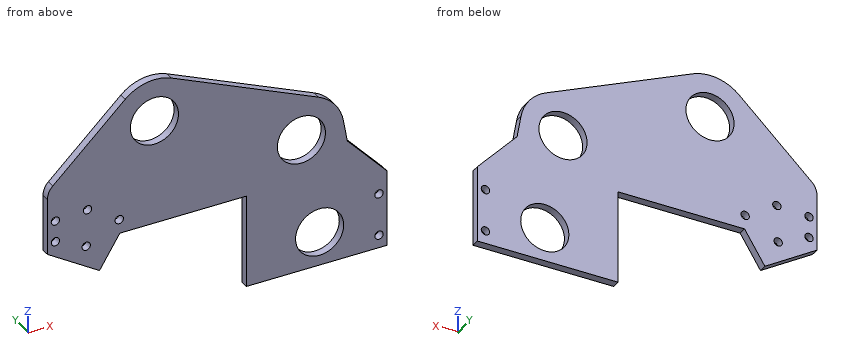
from build123d import *

# Parameters (mm, degrees)
SKETCH1_R              = 14.29004
BOSS_EXTRUDE1_DEPTH    = 4.7625
FILLET1_R              = 10
F_10_CLEARANCE_HOLE1_D = 4.9784
F_10_CLEARANCE_HOLE2_D = 4.9784


with BuildPart() as part:
    # Sketch1 → Boss-Extrude1 (new body)
    with BuildSketch(Plane(origin=(0, 0, 0), x_dir=(1, 0, 0), z_dir=(0, 1, 0))):
        with BuildLine():
            Line((-62.06952, -79.895280222), (25.163028109, -41.695780276))
            ThreePointArc((25.163028109, -41.695780276), (34.911191298, -34.148496119), (39.936134607, -22.890693115))
            Line((39.936134607, -22.890693115), (42.271095404, -9.586739751))
            Line((42.271095404, -9.586739751), (65.82695514, 16.012754812))
            Line((65.82695514, 16.012754812), (65.826833771, 61.726825209))
            Line((65.826833771, 61.726825209), (-17.734439664, 61.726825209))
            Line((-17.734439664, 61.726825209), (-17.734439664, 6.164245545))
            Line((-17.734439664, 6.164245545), (-92.776319002, 6.164245545))
            Line((-92.776319002, 6.164245545), (-104.854054452, 25.49254843))
            Line((-104.854054452, 25.49254843), (-135.785609254, 6.16425364))
            Line((-135.785609254, 6.16425364), (-135.785609254, -31.935712293))
            Line((-135.785609254, -31.935712293), (-89.620113812, -75.16814328))
            ThreePointArc((-89.620113812, -75.16814328), (-76.553580444, -81.662511553), (-62.06952, -79.895280222))
        make_face()
        with Locations(Location((25.821833771, 41.412625209, 0), (0, 0, 90))):
            Circle(SKETCH1_R, mode=Mode.SUBTRACT)
        with Locations(Location((15.012562201, -18.516537909, 0), (0, 0, 90))):
            Circle(SKETCH1_R, mode=Mode.SUBTRACT)
        with Locations(Location((-72.258332946, -56.628468385, 0), (0, 0, 90))):
            Circle(SKETCH1_R, mode=Mode.SUBTRACT)
    extrude(amount=BOSS_EXTRUDE1_DEPTH)

    # Fillet1
    fillet1_edges = [part.edges().sort_by_distance(p)[0] for p in [
        (-135.785609254, 2.38125, 31.935712293),
    ]]
    fillet(fillet1_edges, radius=FILLET1_R)

    # #10 Clearance Hole1 (through all)
    with Locations(Plane(origin=(0, 4.7625, 0), x_dir=(1, 0, 0), z_dir=(0, 1, 0))):
        with Locations((61.064354133, 54.057452946), (61.064421422, 28.712718776), (-131.023109254, -0.185754455), (-131.023109254, -12.885754455)):
            Hole(F_10_CLEARANCE_HOLE1_D / 2)

    # #10 Clearance Hole2 (through all)
    with Locations(Plane(origin=(0, 4.7625, 0), x_dir=(1, 0, 0), z_dir=(0, 1, 0))):
        with Locations((-111.967266406, -14.051352939), (-93.119428737, -2.273847251), (-112.732572492, 8.143472036)):
            Hole(F_10_CLEARANCE_HOLE2_D / 2)


solid = part.part
Source: CAD feature listing. Evaluate the final solid. Frame: model axes, mm. Give positions to 0.01 mm unless a question says otherwise; leave off trailing zeros. Write each loop counter-clockwise with the first axis right and the second up, starting at its lowest first coordinate (ties: lowest second). Pieces come first, ordered by that corner, then holes. Notation, with made-up numbers: M 43,63.25 L 99,63.25 A20 cw 99,86.25 Z; hole C 61.25,41.5 d10. An arc over 180 degrees is marked long. Return JSON: item names as keys, results as strings. Group by question number.
1) Cut plane B-B, the plane z = 44.5. Output: boundary loops of the cut face in (x, y).
2) Cut plane D-D, the plane x = -6.5. Output: boundary loops of the cut face in (y, z).
3) Cut plane A-A, the plane x = -69.5. Output: boundary loops of the cut face in (y, z).
4) Cut plane C-C, the plane y = 3.9. Give the number of separate pieces and of enclosed holes in the cut face, plus the area to 3 significant figures.
5) Pin query (flat end, axial travel): P1, Ø1.4, axis at y = 3, z = -33, coming from the -X side; P2, Ø2.5, axis at x = -39, y = 2, coming from the -Z side; P3, Ø4.5, axis at x = -131.02, z = 0.19, coming from the +Y side; P4, Ø1.5, axis at y = 2, z = -19, coming from the -X side. Return the tip coordinate at first contact, or that it passes through.
6) Material intervals for line 1 along X through (y, z) = (3.35, 12.5); line 2 along X through (y, z) = (2.9, 14); line 3 along Z through (x, y) = (19.5, 1.35), sorted ascending. Write a range as [from, to].
Recorded:
{
 "1": {"outline": "M -122.37,0 L -79.82,0 L -79.82,4.76 L -122.37,4.76 Z; M -64.7,0 L 18.76,0 L 18.76,4.76 L -64.7,4.76 Z"},
 "2": {"outline": "M 0,-61.73 L 4.76,-61.73 L 4.76,55.56 L 0,55.56 Z"},
 "3": {"outline": "M 0,-6.16 L 4.76,-6.16 L 4.76,42.61 L 0,42.61 Z; M 0,70.65 L 4.76,70.65 L 4.76,81.88 L 0,81.88 Z"},
 "4": {"separate pieces": "1", "enclosed holes": "10", "area": "14,700 mm²"},
 "5": {"P1": "stops at x = -17.73", "P2": "stops at z = -6.16", "P3": "passes through", "P4": "stops at x = -116.44"},
 "6": {"line 1": "x = [-135.79, -133.48], [-128.56, -113.91], [-110.02, 2.05], [27.97, 41.76]", "line 2": "x = [-135.79, -133.25], [-128.8, -114.46], [-109.48, 1.46], [28.57, 41.5]", "line 3": "z = [-61.73, -54.23], [-28.6, 4.95], [32.08, 44.18]"}
}
